Source: CAD feature listing. Evaluate the final solid. Frame: model axes, mm. A direction names the side the tool comes from. Round coordinates to 2 decimals unless told otherwise and drop trailing zeros. Loops run counter-clockwise (first coordinate to the right, second up) from the corner with the lowest first, then second, coordinate; pieces in that order, holes last. Notation, with made-up numbers: (-20.75, 71) -> (26.25, 71) arc R24 cw to (26.25, 86) -> close; hole circle Ø2 at (54.5, -26). An arc over 180 degrees is marked (long way). Put each result on its own line as item: value. Start each with the question number.
1. Cut plane A-A (y = 0). Return the cut outline in (x, z), then the cut area to 3 significant figures.
2. Material intervals for L1, parallel to X at y = 13.5, z = 3.1; L2, parallel to X at y = 13, z = 2.8; L3, parallel to Y at x = 10, z = 3.2, sorted ascending.
3. Set-up query: faces 4 (the cylindrical face through (-6.75, -0.03, 2.59)), 5 (the cylindrical face through (-0.17, 1.26, 0.3)). Return all of +Z, -Z, +X, -X, +Y, -Y with unobstructed straight access to the full face (end or side cutting, diameter ignored); none if empty.
4. Contact query for a flat-ended pin moving along its axis: pin 1 (17 mm diameter, centred on x = 0, y = 0, fed in from +Z). Output: stop coordinate, or through.
5. Draft query along Y for faces 1 (the flat face through (10.86, -5.87, 2.59)), 2 (the flat face through (-7, 0, 3.556)), 3 (the flat face through (-5.75, 10.77, 2.59)). Return one class per face: pulls with the +Y half, pulls with the -Y half, needs draft (parallel to the pull), parting line crosses it, or undercut.
Autodesk Inventor part; units mm, degrees
ref_plane "YZ Plane" through (0, 0, 0) normal (1, 0, 0) x (0, 1, 0)
ref_plane "XZ Plane" through (0, 0, 0) normal (0, 1, 0) x (-1, 0, 0)
ref_plane "XY Plane" through (0, 0, 0) normal (0, 0, 1) x (1, 0, 0)
sketch "Sketch1" plane through (0, 0, 0) normal (0, 0, 1) x (1, 0, 0)
  circle A0 centre (0, 0) radius 31.5468
  dimension "d0" = 63.0936
extrude "Extrusion1" add sketch "Sketch1" along normal blind 3.556
sketch "Sketch5" plane through (0, 0, 3.556) normal (0, 0, 1) x (1, 0, 0)
  arc A0 (1.5256, -7.6067) -> (-1.5256, -7.6067) centre (0, -8.5367) ccw
  line L0 (1.5256, -7.6067) -> (10.0877, -14.0155)
  arc A1 (10.0877, -14.0155) -> (14.0155, -10.0877) centre (11.7691, -11.7691) ccw
  line L1 (14.0155, -10.0877) -> (7.6067, -1.5256)
  arc A2 (7.6067, 1.5256) -> (7.6067, -1.5256) centre (8.5367, 0) ccw
  line L2 (7.6067, 1.5256) -> (14.0155, 10.0877)
  arc A3 (14.0155, 10.0877) -> (10.0877, 14.0155) centre (11.7691, 11.7691) ccw
  line L3 (10.0877, 14.0155) -> (1.5256, 7.6067)
  arc A4 (-1.5256, 7.6067) -> (1.5256, 7.6067) centre (0, 8.5367) ccw
  line L4 (-1.5256, 7.6067) -> (-10.0877, 14.0155)
  arc A5 (-10.0877, 14.0155) -> (-14.0155, 10.0877) centre (-11.7691, 11.7691) ccw
  line L5 (-14.0155, 10.0877) -> (-7.6067, 1.5256)
  arc A6 (-7.6067, -1.5256) -> (-7.6067, 1.5256) centre (-8.5367, 0) ccw
  line L6 (-7.6067, -1.5256) -> (-14.0155, -10.0877)
  arc A7 (-14.0155, -10.0877) -> (-10.0877, -14.0155) centre (-11.7691, -11.7691) ccw
  line L7 (-10.0877, -14.0155) -> (-1.5256, -7.6067)
  circle A8 centre (12.339, -12.339) radius 0.75
  circle A9 centre (9.8641, -9.8641) radius 0.75
  circle A10 centre (7.3893, -7.3893) radius 0.75
  circle A11 centre (4.9144, -4.9144) radius 0.75
  circle A12 centre (12.339, 12.339) radius 0.75
  circle A13 centre (9.8641, 9.8641) radius 0.75
  circle A14 centre (7.3893, 7.3893) radius 0.75
  circle A15 centre (4.9144, 4.9144) radius 0.75
  circle A16 centre (-12.339, 12.339) radius 0.75
  circle A17 centre (-9.8641, 9.8641) radius 0.75
  circle A18 centre (-7.3893, 7.3893) radius 0.75
  circle A19 centre (-4.9144, 4.9144) radius 0.75
  circle A20 centre (-12.339, -12.339) radius 0.75
  circle A21 centre (-9.8641, -9.8641) radius 0.75
  circle A22 centre (-7.3893, -7.3893) radius 0.75
  circle A23 centre (-4.9144, -4.9144) radius 0.75
  circle A24 centre (0, 0) radius 3.6
extrude "Extrusion4" cut sketch "Sketch5" against normal blind 1.9558 contours A0 L7 A7 L6 A6 L5 A5 L4 A4 L3 A3 L2 A2 L1 A1 L0 | A8 | A9 | A10 | A11 | A12 | A13 | A14 | A15 | A16 | A17 | A18 | A19 | A20 | A21 | A22 | A23 | A24
sketch "Sketch6" plane through (0, 0, 0) normal (0, 1, 0) x (-1, 0, 0)
  point P0 (0, 0)
sketch "Sketch7" plane through (0, 0, 0) normal (0, 1, 0) x (-1, 0, 0)
  point P0 (0, 0)
sketch "Sketch8" plane through (0, 0, 0) normal (1, 0, 0) x (0, 1, 0)
  line L0 (31.5468, 0) -> (31.5468, 3.556)
  circle A0 centre (31.5468, 1.778) radius 1.7361
  line L1 (0, 0) -> (0, 3.556)
  line L2 (31.5468, 3.556) -> (-31.5468, 3.556)
revolve "Revolution1" cut sketch "Sketch8" angle 360 about axis through (0, 0, 0) along (0, 0, 1)
sketch "Sketch9" plane through (0, 0, 1.6002) normal (0, 0, 1) x (1, 0, 0)
  circle A0 centre (0, 0) radius 1.27
  circle A1 centre (0, 0) radius 5.2705
extrude "Extrusion5" cut sketch "Sketch9" along normal mid plane 25.4 contours A0
sketch "Sketch10" plane through (0, 0, 3.556) normal (0, 0, 1) x (1, 0, 0)
  point P0 (0, 0)
sketch "Sketch11" plane through (0, 0, 1.6002) normal (0, 0, 1) x (1, 0, 0)
  circle A0 centre (0, 0) radius 5.2705
extrude "Extrusion6" cut sketch "Sketch11" against normal blind 1.016
properties part number "Aidan Sherry Wheel"
Solution:
1. outline: (-31.55, 0) -> (-1.27, 0) -> (-1.27, 0.58) -> (-5.27, 0.58) -> (-5.27, 1.6) -> (-6.75, 1.6) -> (-6.75, 3.56) -> (-31.55, 3.56) -> (-31.55, 3.51) arc R1.74 cw to (-31.55, 0.04) -> close; (1.27, 0) -> (31.55, 0) -> (31.55, 0.04) arc R1.74 cw to (31.55, 3.51) -> (31.55, 3.56) -> (6.75, 3.56) -> (6.75, 1.6) -> (5.27, 1.6) -> (5.27, 0.58) -> (1.27, 0.58) -> close
1. area: 176 mm^2
2. L1: x = -27.26 to -13.98, -9.4 to 9.4, 13.98 to 27.26
2. L2: x = -27.2 to -14.29, -8.73 to 8.73, 14.29 to 27.2
2. L3: y = -28.87 to -13.95, -4.72 to 4.72, 13.95 to 28.87
3. face 4: +Z
3. face 5: +Z, -Z
4. pin 1: stops at z = 3.56
5. face 1: undercut
5. face 2: needs draft
5. face 3: undercut
